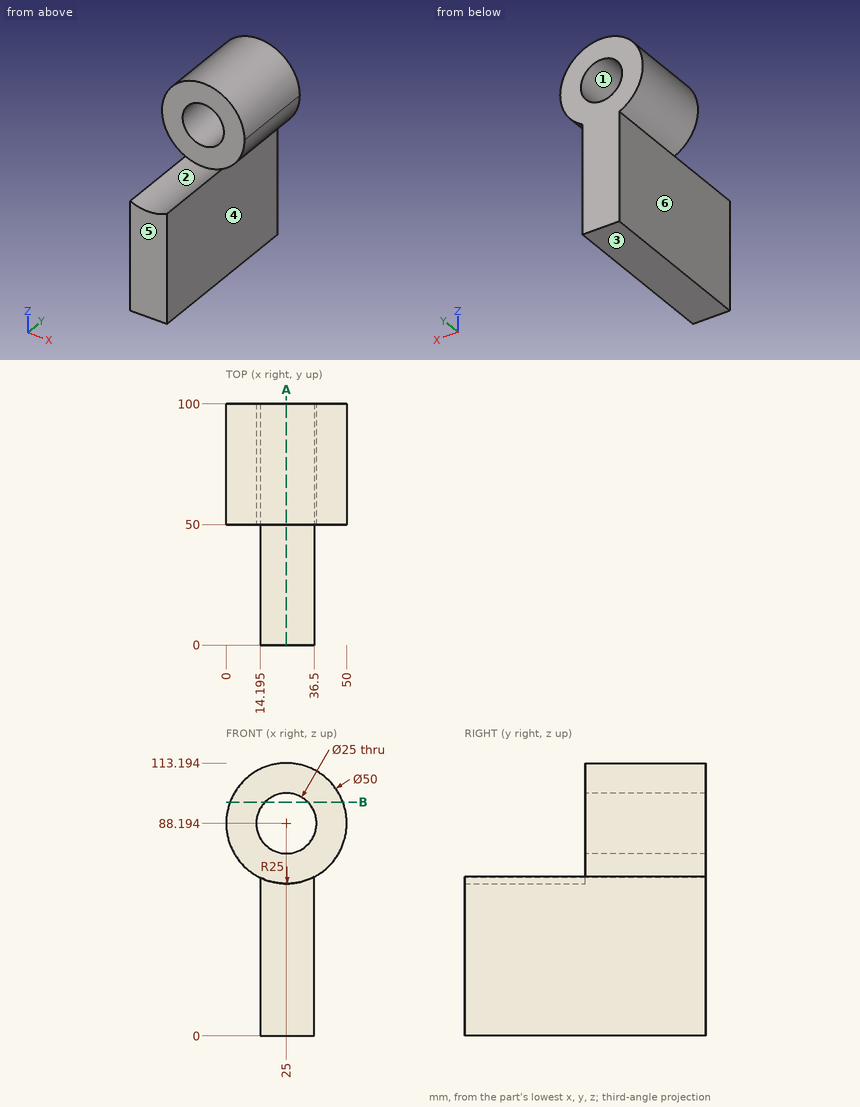
The figure shows three views and two pictorial views of one solid part (mm, origin at its lowest corner). Answer the questions. A direction names the side the tool comes from. Coordinates: 2 decimals unless noted, no trailing zeros. Loops run counter-clockwise (first coordinate to the right, second up) from the corner with the lowest first, then second, coordinate; pieces in that order, holes last. Notation, with made-up numbers: (-12.5, -30) -> (26.5, -30) arc R19 ccw to (26.5, -1) -> close; hole circle Ø2 at (42, 66). An arc over 180 degrees is marked (long way). Return JSON: item names as keys, results as strings. Group by question number.
(1) Which of the six approach directions +Z, -Z, +X, -X, +Y, -Y give full straight-line access (tool end or side, diameter ignored) to the marked faces 5 and 6?
(2) A cutting plane is placed at B-B on z = 97. Write down the section's boundary in (x, y).
(3) Given pin 1 Ø8 at (x, y) = (29.5, 11.5) entering from +Z; pin 2 Ø4 at (y, z) = (79.5, 32.5) entering from -X (1 decimal); pin 3 Ø2 at (x, y) = (44, 69.5) entering from -Z (1 decimal), each flat-ended and moving along its own axis, determine where each tip first touches the part or whether it passes through.
(4) A cutting plane is placed at A-A on x = 25. Write down the section's boundary in (y, z), and give its area (3 significant figures).
(5) Find the intervals of material crossed by probe 1 along Z at (x, y) = (25, 70); probe 2 along X at (y, z) = (39, 63) (1 decimal); probe 3 along Y at (x, z) = (36, 70), in increasing order. Write a range as from..to.
(6) Determine the mould class of the marked faces 1, 2, 3 and 4 for opening direction X: released by +X, released by -X, zero draft, split by the parting line, or undercut.
The answers:
{
 "1": {"face 5": "+Z, -Z, +X, -X, -Y", "face 6": "-Z, -X, +Y, -Y"},
 "2": {"outline": "(1.6, 50) -> (16.13, 50) -> (16.13, 100) -> (1.6, 100) -> close; (33.87, 50) -> (48.4, 50) -> (48.4, 100) -> (33.87, 100) -> close"},
 "3": {"pin 1": "stops at z = 64.68", "pin 2": "stops at x = 14.2", "pin 3": "stops at z = 70.8"},
 "4": {"outline": "(0, 0) -> (100, 0) -> (100, 75.69) -> (50, 75.69) -> (50, 63.19) -> (0, 63.19) -> close; (50, 100.69) -> (100, 100.69) -> (100, 113.19) -> (50, 113.19) -> close", "area": "7,570 mm^2"},
 "5": {"probe 1": "z = 0..75.69, 100.69..113.19", "probe 2": "x = 14.2..36.5", "probe 3": "y = 50..100"},
 "6": {"face 1": "undercut", "face 2": "undercut", "face 3": "zero draft", "face 4": "released by +X"}
}
